Can you work these out from the model? Positions are in its coordinate system, mm. Face numbers are marked on the shaded views. A direction names the side the tool comes from. Round coordinates to 2 decimals unless told otherwise and drop trailing zeros. Loops run counter-clockwise (first coordinate to the right, second up) from the corner with the lowest first, then second, coordinate; pieces in that order, holes last. Notation, with made-up numbers: (50.5, -28.5) -> (94.5, -28.5) arc R20 ccw to (94.5, 8.5) -> close; hole circle Ø8 at (-39.75, 1.25). An arc over 180 degrees is marked (long way). Write item = value, one per line.
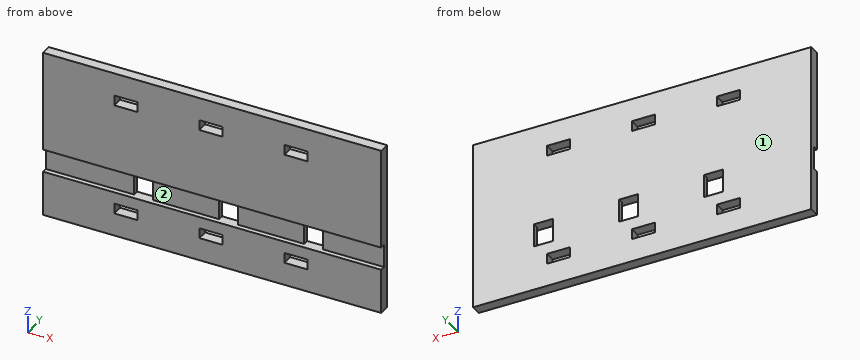
from build123d import *

# Parameters (mm, degrees)
SKETCH1_W                     = 101.092
SKETCH1_H                     = 50.292
BOSS_EXTRUDE1_DEPTH           = 3.175
SKETCH2_W                     = 5.588
SKETCH2_H                     = 6.858
WIRE_HOLE_DEPTH               = 4.175
SKETCH3_W                     = 6.858
SKETCH3_H                     = 3.048
CUT_EXTRUDE2_DEPTH            = 4.175
LPATTERN1_COUNT               = 2
LPATTERN1_PITCH               = 25.4
LPATTERN1_COPY_1_SKETCH_W     = 6.858
LPATTERN1_COPY_1_SKETCH_H     = 3.048
LPATTERN1_COPY_1_DEPTH        = 4.175
LPATTERN1_COL_COUNT           = 2
LPATTERN1_COL_PITCH           = 25.4
LPATTERN1_COL_COPY_1_SKETCH_W = 6.858
LPATTERN1_COL_COPY_1_SKETCH_H = 3.048
LPATTERN1_COL_COPY_1_DEPTH    = 4.175
SKETCH4_W                     = 101.092
SKETCH4_H                     = 6.858
CUT_EXTRUDE3_DEPTH            = 1.524


with BuildPart() as part:
    # Sketch1 → Boss-Extrude1 (new body)
    with BuildSketch(Plane(origin=(0, 0, 0), x_dir=(1, 0, 0), z_dir=(0, 1, 0))):
        Rectangle(SKETCH1_W, SKETCH1_H)
    extrude(amount=BOSS_EXTRUDE1_DEPTH)

    # Sketch2 → Wire Hole (cut, through all)
    with BuildSketch(Plane(origin=(0, 3.175, 0), x_dir=(1, 0, 0), z_dir=(0, 1, 0))):
        with Locations((4.064, 8.322545685)):
            Rectangle(SKETCH2_W, SKETCH2_H)
    wire_hole = extrude(amount=-WIRE_HOLE_DEPTH, mode=Mode.SUBTRACT)

    # Sketch3 → Cut-Extrude2 (cut, through all)
    with BuildSketch(Plane(origin=(0, 3.175, 0), x_dir=(1, 0, 0), z_dir=(0, 1, 0))):
        with Locations((-0.381, 16.764)):
            Rectangle(SKETCH3_W, SKETCH3_H)
    cut_extrude2 = extrude(amount=-CUT_EXTRUDE2_DEPTH, mode=Mode.SUBTRACT)

    # Mirror1: Cut-Extrude2 across plane
    add(cut_extrude2.mirror(Plane.XY), mode=Mode.SUBTRACT)

    # LPattern1: Wire Hole, Cut-Extrude2 ×2
    with Locations(*[(-i * LPATTERN1_PITCH, 0, 0) for i in range(1, LPATTERN1_COUNT)]):
        add(wire_hole, mode=Mode.SUBTRACT)
        add(cut_extrude2, mode=Mode.SUBTRACT)

    # LPattern1 copy 1 sketch → LPattern1 copy 1 (cut, through all)
    with BuildSketch(Plane(origin=(-25.4, 3.175, 0), x_dir=(1, 0, 0), z_dir=(0, 1, 0))):
        with Locations((-0.381, -16.764)):
            Rectangle(LPATTERN1_COPY_1_SKETCH_W, LPATTERN1_COPY_1_SKETCH_H)
    extrude(amount=-LPATTERN1_COPY_1_DEPTH, mode=Mode.SUBTRACT)

    # LPattern1 col: Wire Hole, Cut-Extrude2 ×2
    with Locations(*[(i * LPATTERN1_COL_PITCH, 0, 0) for i in range(1, LPATTERN1_COL_COUNT)]):
        add(wire_hole, mode=Mode.SUBTRACT)
        add(cut_extrude2, mode=Mode.SUBTRACT)

    # LPattern1 col copy 1 sketch → LPattern1 col copy 1 (cut, through all)
    with BuildSketch(Plane(origin=(25.4, 3.175, 0), x_dir=(1, 0, 0), z_dir=(0, 1, 0))):
        with Locations((-0.381, -16.764)):
            Rectangle(LPATTERN1_COL_COPY_1_SKETCH_W, LPATTERN1_COL_COPY_1_SKETCH_H)
    extrude(amount=-LPATTERN1_COL_COPY_1_DEPTH, mode=Mode.SUBTRACT)

    # Sketch4 → Cut-Extrude3 (cut)
    with BuildSketch(Plane(origin=(0, 0, 0), x_dir=(1, 0, 0), z_dir=(0, 1, 0))):
        with Locations((0, 8.322545685)):
            Rectangle(SKETCH4_W, SKETCH4_H)
    extrude(amount=CUT_EXTRUDE3_DEPTH, mode=Mode.SUBTRACT)


solid = part.part
1. Suppose I cut it at A-A, the plane x = -1. List the corners of the cut face in (y, z) for me (3 decimals).
Entries:
outline = (0, -25.146) -> (3.175, -25.146) -> (3.175, -18.288) -> (0, -18.288) -> close; (0, -15.24) -> (3.175, -15.24) -> (3.175, 15.24) -> (0, 15.24) -> (0, -4.894) -> (1.524, -4.894) -> (1.524, -11.752) -> (0, -11.752) -> close; (0, 18.288) -> (3.175, 18.288) -> (3.175, 25.146) -> (0, 25.146) -> close
2. Suppose I cut it at B-B, the plane y = 0.5. Count the separate pieces of the cut face and the enclosed holes in it, and give its area (3 significant figures).
Entries:
separate_pieces = 2
enclosed_holes = 6
area = 4,270 mm²
3. I need wall thicknesses on line 1 (Z direction, x = -27.5, y = 1.95); line 2 (Z direction, x = 26.5, y = 0.55); line 3 (X direction, y = 1.8, z = 17). Which ranges of each line are inside material? Lowest first, please. Write a range as [from, to].
Entries:
line_1 = [-25.15, -18.29], [-15.24, 15.24], [18.29, 25.15]
line_2 = [-25.15, -18.29], [-15.24, -11.75], [-4.89, 15.24], [18.29, 25.15]
line_3 = [-50.55, -29.21], [-22.35, -3.81], [3.05, 21.59], [28.45, 50.55]
4. Suppose I cut it at C-C, the plane x = 31. List the corners of the cut face in (y, z) for me (3 decimals), and give its area (3 significant figures).
Entries:
outline = (0, -25.146) -> (3.175, -25.146) -> (3.175, -11.752) -> (0, -11.752) -> close; (0, -4.894) -> (3.175, -4.894) -> (3.175, 25.146) -> (0, 25.146) -> close
area = 138 mm²
5. Suppose I cut it at D-D, the plane x = -42.5. List the corners of the cut face in (y, z) for me (3 decimals), and give its area (3 significant figures).
Entries:
outline = (0, -25.146) -> (3.175, -25.146) -> (3.175, 25.146) -> (0, 25.146) -> (0, -4.894) -> (1.524, -4.894) -> (1.524, -11.752) -> (0, -11.752) -> close
area = 149 mm²
6. For the marked faces 1 and 2, which set-ups out of +Z, -Z, +X, -X, +Y, -Y let a thin tool reach every point of the face, with its end or its side?
Entries:
face_1 = +Z, -Z, +X, -X, +Y
face_2 = +X, -X, -Y
